from build123d import *

# Parameters (mm, degrees)
CROQUIS1_R              = 7.6
CROQUIS1_R_2            = 6.6
SALIENTE_EXTRUIR1_DEPTH = 5
CROQUIS3_R              = 9.6
CROQUIS3_R_2            = 7.6
CROQUIS3_R_3            = 6.6
CROQUIS3_R_4            = 5
SALIENTE_EXTRUIR2_DEPTH = 1
BOSS_EXTRUDE1_START     = -6
CROQUIS3_4_R            = 9.6
CROQUIS3_4_R_2          = 7.6
CROQUIS3_4_R_3          = 6.6
BOSS_EXTRUDE1_DEPTH     = 1
REDONDEO1_R             = 2


with BuildPart() as part:
    # Croquis1 → Saliente-Extruir1 (new body)
    with BuildSketch(Plane.XY):
        Circle(CROQUIS1_R)
        Circle(CROQUIS1_R_2, mode=Mode.SUBTRACT)
    extrude(amount=SALIENTE_EXTRUIR1_DEPTH)

    # Croquis3 → Saliente-Extruir2 (add)
    # profile 1 of 3: a face of its own
    with BuildSketch(Plane.XY.offset(5)):
        Circle(CROQUIS3_R)
        Circle(CROQUIS3_R_2, mode=Mode.SUBTRACT)
    # profile 2 of 3: a face of its own
    with BuildSketch(Plane.XY.offset(5)):
        Circle(CROQUIS3_R_2)
        Circle(CROQUIS3_R_3, mode=Mode.SUBTRACT)
    # profile 3 of 3: a face of its own
    with BuildSketch(Plane.XY.offset(5)):
        Circle(CROQUIS3_R_3)
        Circle(CROQUIS3_R_4, mode=Mode.SUBTRACT)
    extrude(amount=SALIENTE_EXTRUIR2_DEPTH)

    # Croquis3<4> → Boss-Extrude1 (add)
    # profile 1 of 2: a face of its own
    with BuildSketch(Plane.XY.offset(5).offset(BOSS_EXTRUDE1_START)):
        Circle(CROQUIS3_4_R)
        Circle(CROQUIS3_4_R_2, mode=Mode.SUBTRACT)
    # profile 2 of 2: a face of its own
    with BuildSketch(Plane.XY.offset(5).offset(BOSS_EXTRUDE1_START)):
        Circle(CROQUIS3_4_R_2)
        Circle(CROQUIS3_4_R_3, mode=Mode.SUBTRACT)
    extrude(amount=BOSS_EXTRUDE1_DEPTH)

    # Redondeo1
    redondeo1_edges = [part.edges().sort_by_distance(p)[0] for p in [
        (-7.6, 0, 0),
        (-7.6, 0, 5),
    ]]
    fillet(redondeo1_edges, radius=REDONDEO1_R - 0.0001)  # a hair under: the kernel refuses the full size


solid = part.part
Could you check a few things on this model? Use its own coordinates, in mm. A direction names the side the tool comes from. Coordinates: 2 decimals unless noted, no trailing zeros. Loops run counter-clockwise (first coordinate to the right, second up) from the corner with the lowest first, then second, coordinate; pieces in that order, holes last.
1. For faces 1 (the face through (-7.593, 0.334, 2.493)), 2 (the face through (-7, -2, -1)), 3 (the face through (-4.864, 4.461, 1.958)), which set-ups out of +Z, -Z, +X, -X, +Y, -Y let a thin tool reach every point of the face, with its end or its side?
2. Imagine slicing it at D-D (z = 4.5). Please give me the cut outline in (x, y).
3. Imagine slicing it at C-C (z = -0.5). Please give me the cut outline in (x, y).
4. For P1, Ø1, axis at x = 1.5, z = 0, coming from the -Y side, with a flat end and sliding along its axis, tell me the tip position at first contact or that it passes through.
5. I need wall thicknesses on L1, parallel to Z at x = -8, y = -5.25; L2, parallel to Y at x = 0, z = 3; L3, parallel to Y at x = -0.5, z = 4. Which ranges of each line are inside material? Lowest first, please.
6. We'd pull the mould along Y, two halves only. Please class faces 4 (the face through (5.161, 8.095, 5.493)), 5 (the face through (4, -4, 6)), 6 (the face through (-3.9, 3.5, 5)): released by +Y, released by -Y, zero draft, split by the parting line, or undercut.
Computed values:
1. face 1: none
1. face 2: -Z, +X, -X, +Y, -Y
1. face 3: -Z
2. outline: circle Ø16.55 at (0, 0); hole circle Ø13.2 at (0, 0)
3. outline: circle Ø19.2 at (0, 0); hole circle Ø13.2 at (0, 0)
4. P1: stops at y = -9.55
5. L1: z = -1 to 0, 5 to 6
5. L2: y = -7.6 to -6.6, 6.6 to 7.6
5. L3: y = -7.85 to -6.58, 6.58 to 7.85
6. face 4: split by the parting line
6. face 5: zero draft
6. face 6: undercut
